```python
from build123d import *

# Parameters (mm, degrees)
F1_DEPTH = 65.43193
F2_R     = 31.223032
F3_DEPTH = 109.98878
F5_DEPTH = 101.69795


with BuildPart() as f1:
    # F0 (on Top) → F1 (new body)
    with BuildSketch(Plane.XY):
        with BuildLine():
            ThreePointArc((-73.905277, -18.434329), (-96.395829, -27.169836), (-83.585647, -47.615697))
            ThreePointArc((-83.585647, -47.615697), (-2.563987, -58.296785), (-73.905277, -18.434329))
        make_face()
    extrude(amount=F1_DEPTH)

    # F2 (on face) → F3 (cut)
    with BuildSketch(Plane.XY.offset(65.43193)):
        with Locations((-42.051967, -45.19739)):
            Circle(F2_R)
    extrude(amount=-F3_DEPTH, mode=Mode.SUBTRACT)

    # F4 (on face) → F5 (cut)
    with BuildSketch(Plane.XY.offset(65.43193)):
        with BuildLine():
            ThreePointArc((-83.611005, -43.263185), (-81.539948, -32.097995), (-76.527057, -21.908703))
            ThreePointArc((-76.527057, -21.908703), (-92.318031, -28.522569), (-83.611005, -43.263185))
        make_face()
    extrude(amount=-F5_DEPTH, mode=Mode.SUBTRACT)


solid = f1.part
```
The model under review builds one solid part; all positions refer to its coordinate system, in mm. Round coordinates to 2 decimals unless told otherwise and drop trailing zeros. Order: outer loops, then holes, each group sorted by start corner. A loop starts at its lowest first (then second) coordinate and runs counter-clockwise, first axis right, second up. Notation, with made-up numbers: (-26.75, -28) - (-11.75, -28) arc R13 ccw to (-11.75, -13) - close; hole circle Ø3 at (-16.75, 78). An arc over 180 degrees is marked (long way). Answer in a Markdown table with one row per item.
(1) Mouldability with a two-part tool opening along X and no side actions: class faces 1 (the face through (-74, -42, 65.432)), 2 (the face through (-81.59, -32.25, 33.17)), 3 (the face through (-92.23, -28.27, 33.17)) as released by +X, released by -X, zero draft, split by the parting line, or undercut.
Result set:
| item | result |
|---|---|
| face 1 | zero draft |
| face 2 | undercut |
| face 3 | undercut |
(2) Clearance check with flat-ended pins moving along their axes: P1, Ø1.5, axis at y = -26, z = 53, coming from the -X side; P2, Ø6, axis at y = -27.5, z = 41, coming from the +X side; P3, Ø1, axis at x = -17.5, z = 40.5, coming from the -Y side; P4, Ø12, axis at x = -62.5, y = -27, coming from the +Z side. State where each tip first meets the part, or that it passes through.
Result set:
| item | result |
|---|---|
| P1 | stops at x = -96.25 |
| P2 | stops at x = -3.13 |
| P3 | stops at y = -79.14 |
| P4 | stops at z = 65.43 |
(3) Take a section at D-D on z = 46. Write out the cut boundary in (x, y).
Result set:
| item | result |
|---|---|
| outline | (-83.59, -47.62) arc R41.6 ccw (long way) to (-73.91, -18.43) arc R15.65 ccw (long way) to start; hole (-83.61, -43.26) arc R41.6 cw to (-76.53, -21.91) arc R11.36 ccw (long way) to start; hole circle Ø62.45 at (-42.05, -45.2) |
(4) Take a section at A-A on y = -39. Write out the cut boundary in (x, z).
Result set:
| item | result |
|---|---|
| outline | (-95.59, 0) - (-90.56, 0) - (-90.56, 65.43) - (-95.59, 65.43) - close; (-83.19, 0) - (-72.65, 0) - (-72.65, 65.43) - (-83.19, 65.43) - close; (-11.45, 0) - (-0.91, 0) - (-0.91, 65.43) - (-11.45, 65.43) - close |
(5) Take a section at B-B on x = -36. Write out the cut boundary in (y, z), plus the area to 3 significant figures.
Result set:
| item | result |
|---|---|
| outline | (-86.36, 0) - (-75.83, 0) - (-75.83, 65.43) - (-86.36, 65.43) - close; (-14.57, 0) - (-4.04, 0) - (-4.04, 65.43) - (-14.57, 65.43) - close |
| area | 1,380 mm2 |
(6) For line 1 (X direction, y = -38.5, z = 49); line 2 (X direction, y = -25, z = 3); line 3 (X direction, y = -73, z = 21), list the stretches that pass through material, from the lowest coordinate up. Write a range as from..to.
Result set:
| item | result |
|---|---|
| line 1 | x = -95.82..-90.92, -83.11..-72.55, -11.56..-0.99 |
| line 2 | x = -95.49..-90.4, -78.42..-65.86, -18.24..-5.68 |
| line 3 | x = -73..-56.26, -27.84..-11.1 |
(7) Take a section at C-C on y = -63.5. Write out the cut boundary in (x, z), plus the area to 3 significant figures.
Result set:
| item | result |
|---|---|
| outline | (-79.41, 0) - (-67.35, 0) - (-67.35, 65.43) - (-79.41, 65.43) - close; (-16.76, 0) - (-4.69, 0) - (-4.69, 65.43) - (-16.76, 65.43) - close |
| area | 1,580 mm2 |
